from build123d import *

# Parameters (mm, degrees)
F0_W         = 33
F0_H         = 14
F0_R         = 1.75
F1_DEPTH     = 4.8
F2_R         = 1.5
F4_DEPTH     = 4.8
F2_W         = 33
F2_H         = 14
F2_R_2       = 2.5
F2_R_3       = 1.75
F5_DEPTH     = 3.5
F7_DEPTH     = 2.5
F8_W         = 6.5
F8_H         = 5.7518341467
F9_DEPTH     = 12.5
F10_R        = 6
F11_T1_DEPTH = 79.0934091739
F12_R        = 2


# Not quite as in the source:
# - a fillet or chamfer that OpenCascade refuses, or shapes differently, is made with other operations: its cross-section is extruded or revolved along the edge and cut away or added


with BuildPart() as f1:
    # F0 (on Top) → F1 (new body)
    with BuildSketch(Plane.XY):
        with Locations((0, 1.2481658533)):
            Rectangle(F0_W, F0_H)
        with Locations((-13.585, 0)):
            Circle(F0_R, mode=Mode.SUBTRACT)
        with Locations((13.585, 0)):
            Circle(F0_R, mode=Mode.SUBTRACT)
    extrude(amount=F1_DEPTH)

    # F2 (on face) → F4 (cut, through all)
    with BuildSketch(Plane.XY.offset(4.8)):
        with Locations((-7.585, -3)):
            Circle(F2_R)
        with Locations((0, 5)):
            Circle(F2_R)
        with Locations((7.585, -3)):
            Circle(F2_R)
    extrude(amount=-F4_DEPTH, mode=Mode.SUBTRACT)

    # F2 (on face) → F5 (cut)
    with BuildSketch(Plane.XY.offset(4.8)):
        with Locations((0, 1.2481658533)):
            Rectangle(F2_W, F2_H)
        with Locations((-7.585, -3)):
            Circle(F2_R_2, mode=Mode.SUBTRACT)
        with Locations((-13.585, 0)):
            Circle(F2_R_3, mode=Mode.SUBTRACT)
        with Locations((7.585, -3)):
            Circle(F2_R_2, mode=Mode.SUBTRACT)
        with Locations((13.585, 0)):
            Circle(F2_R_3, mode=Mode.SUBTRACT)
        with Locations((0, 5)):
            Circle(F2_R_2, mode=Mode.SUBTRACT)
    extrude(amount=-F5_DEPTH, mode=Mode.SUBTRACT)

    # F6: chamfer of 4 x 2 on 3 edges, made by hand


with BuildPart() as f6_tool2:
    # F6_s3 → F6_t4 (revolve)
    with BuildSketch(Plane.XZ.offset(3)):
        Polygon((-3.085, 1.3), (-5.085, 5.3), (-5.085, 1.3), align=None)
    revolve(axis=Axis((-7.585, -3, 1.3), (0, 0, 1)))

    split(bisect_by=Plane.XZ.offset(5.7518341467), keep=Keep.BOTTOM)

    split(bisect_by=Plane.XY.offset(4.8), keep=Keep.BOTTOM)


with BuildPart() as f1_1:
    add(f1.part)

    # F6_t1: union F6_tool2
    add(f6_tool2.part)


with BuildPart() as f6_tool8:
    # F6_s9 → F6_t10 (revolve)
    with BuildSketch(Plane.XZ.offset(-5)):
        Polygon((4.5, 1.3), (2.5, 5.3), (2.5, 1.3), align=None)
    revolve(axis=Axis((0, 5, 1.3), (0, 0, 1)))

    split(bisect_by=Plane.XZ.offset(-8.2481658533), keep=Keep.TOP)

    split(bisect_by=Plane.XY.offset(4.8), keep=Keep.BOTTOM)


with BuildPart() as f1_2:
    add(f1_1.part)

    # F6_t7: union F6_tool8
    add(f6_tool8.part)


with BuildPart() as f6_tool14:
    # F6_s15 → F6_t16 (revolve)
    with BuildSketch(Plane.XZ.offset(3)):
        Polygon((12.085, 1.3), (10.085, 5.3), (10.085, 1.3), align=None)
    revolve(axis=Axis((7.585, -3, 1.3), (0, 0, 1)))

    split(bisect_by=Plane.XZ.offset(5.7518341467), keep=Keep.BOTTOM)

    split(bisect_by=Plane.XY.offset(4.8), keep=Keep.BOTTOM)


with BuildPart() as f1_3:
    add(f1_2.part)

    # F6_t13: union F6_tool14
    add(f6_tool14.part)

    # F3 (on face) → F7 (cut)
    with BuildSketch(Plane(origin=(0, 0, 0), x_dir=(1, 0, 0), z_dir=(0, 0, -1))):
        Polygon((-5.8818167059, 5.95), (-9.2881832941, 5.95), (-9.4025944029, 5.7518341467), (-5.7674055971, 5.7518341467), align=None)
        Polygon((9.4025944029, 5.7518341467), (5.7674055971, 5.7518341467), (4.1786334118, 3), (5.8818167059, 0.05), (9.2881832941, 0.05), (10.9913665882, 3), align=None)
        Polygon((-1.7031832941, -7.95), (1.7031832941, -7.95), (3.4063665882, -5), (1.7031832941, -2.05), (-1.7031832941, -2.05), (-3.4063665882, -5), align=None)
        Polygon((-5.7674055971, 5.7518341467), (-9.4025944029, 5.7518341467), (-10.9913665882, 3), (-9.2881832941, 0.05), (-5.8818167059, 0.05), (-4.1786334118, 3), align=None)
    extrude(amount=-F7_DEPTH, mode=Mode.SUBTRACT)

    # F8 (on face) → F9 (cut, symmetric)
    with BuildSketch(Plane.XY.offset(1.3)):
        with Locations((-0.835, -2.8759170733)):
            Rectangle(F8_W, F8_H)
    extrude(amount=F9_DEPTH, both=True, mode=Mode.SUBTRACT)

    # F10
    f10_edges = [f1_3.edges().sort_by_distance(p)[0] for p in [
        (-16.5, -5.751834, 0.65),
        (16.5, -5.751834, 0.65),
    ]]
    fillet(f10_edges, radius=F10_R)

    # F11: chamfer of 6 x 15 on 2 edges, made by hand

    # F11_s2 → F11_t1 (cut)
    with BuildSketch(Plane.XY.offset(-38.896704587)):
        Polygon((-1.5, 8.2481658533), (-16.5, 2.2481658533), (-16.5, 8.2481658533), align=None)
        Polygon((16.5, 2.2481658533), (1.5, 8.2481658533), (16.5, 8.2481658533), align=None)
    extrude(amount=F11_T1_DEPTH, mode=Mode.SUBTRACT)

    # F12 (call 1 of 5: OpenCascade refuses the feature's edges together)
    f12_edges = [f1_3.edges().sort_by_distance(p)[0] for p in [
        (-4.085, 0, 0.65),
    ]]
    fillet(f12_edges, radius=F12_R)

    # F12#2 (call 2 of 5)
    f12_2_edges = [f1_3.edges().sort_by_distance(p)[0] for p in [
        (2.415, 0, 0.65),
    ]]
    fillet(f12_2_edges, radius=F12_R)

    # F12#3 (call 3 of 5)
    f12_3_edges = [f1_3.edges().sort_by_distance(p)[0] for p in [
        (2.415, -5.751834, 0.65),
    ]]
    fillet(f12_3_edges, radius=F12_R)

    # F12#4 (call 4 of 5)
    f12_4_edges = [f1_3.edges().sort_by_distance(p)[0] for p in [
        (16.5, 2.248166, 0.65),
    ]]
    fillet(f12_4_edges, radius=F12_R)

    # F12#5 (call 5 of 5)
    f12_5_edges = [f1_3.edges().sort_by_distance(p)[0] for p in [
        (-16.5, 2.248166, 0.65),
    ]]
    fillet(f12_5_edges, radius=F12_R)


solid = f1_3.part
Could you check a few things on this model? Use its own coordinates, in mm. A direction names the side the tool comes from. Give positions to 0.01 mm unless a question says otherwise; leave off trailing zeros. Loops run counter-clockwise (first coordinate to the right, second up) from the corner with the lowest first, then second, coordinate; pieces in that order, holes last. Notation, with made-up numbers: (-11, 56) -> (10, 56) arc R10 cw to (10, 72) -> close; hole circle Ø7 at (5, 17). An arc over 180 degrees is marked (long way). Return JSON: item names as keys, results as strings.
Item 1: If we section it at B-B on z = 0.3: Count the separate pieces of the cut face and the enclosed holes in it, plus the area to 3 significant figures.
Geometry results:
{"separate pieces": "1", "enclosed holes": "3", "area": "211 mm²"}
Item 2: If we section it at A-A on x = 0: List the corners of the cut face in (y, z) for me, plus the area to 3 significant figures.
Geometry results:
{"outline": "(0, 0) -> (2.05, 0) -> (2.05, 2.5) -> (3.5, 2.5) -> (3.5, 4.8) -> (2.25, 4.8) -> (0.5, 1.3) -> (0, 1.3) -> close; (6.5, 2.5) -> (7.95, 2.5) -> (7.95, 0) -> (8.25, 0) -> (8.25, 3.8) -> (7.75, 4.8) -> (6.5, 4.8) -> close", "area": "12.9 mm²"}
Item 3: If we section it at C-C on x = 13: List the corners of the cut face in (y, z) for me, plus the area to 3 significant figures.
Geometry results:
{"outline": "(-5.21, 0) -> (-1.65, 0) -> (-1.65, 1.3) -> (-5.21, 1.3) -> close; (1.65, 0) -> (3.65, 0) -> (3.65, 1.3) -> (1.65, 1.3) -> close", "area": "7.22 mm²"}
Item 4: We'd pull the mould along X, two halves only. Please class faces 4 (the flat face through (0, 7.95, 1)), 5 (the flat face through (8.47, 5.46, 0.85)), 6 (the flat face through (-8.275, 5.538, 0.851)): +X half, -X half, draft (parallel to the pull), parting line (faces both ways), or undercut.
Geometry results:
{"face 4": "undercut", "face 5": "+X half", "face 6": "-X half"}
Item 5: I'm going to push flat-ended pins straight in: pin 1 (1 mm diameter, centred on x = 5, z = 1.5, fed in from +Y); pin 2 (0.6 mm diameter, centred on x = -1.5, z = 0.5, fed in from -Y); pin 3 (2 mm diameter, centred on y = 4, z = 3, fed in from +X). Where does each tip first touch, or does it pass through?
Geometry results:
{"pin 1": "stops at y = 7.03", "pin 2": "stops at y = 0", "pin 3": "stops at x = 4.07"}
Item 6: Which directions (+Z, -Z, +X, -X, +Y, -Y) give clear straight access to the entire face, cutting with the end or side of a thin tool? Please do faces 1 (the flat face through (4.984, -4.395, 1.232)), 2 (the flat face through (2.415, -3, 1)), 3 (the flat face through (-8, -0.05, 1)).
Geometry results:
{"face 1": "-Z", "face 2": "+Z, -Z, -Y", "face 3": "-Z, -Y"}
Item 7: I need wall thicknesses on L1, parallel to X at y = -4, z = 0.3 (3 decimals); L2, parallel to X at y = -2.5, z = 2.65 (3 decimals); L3, parallel to Z at x = -6.5, y = 4.75. Which ranges of each line are inside material? Lowest first, please. Write a range as from..to.
Geometry results:
{"L1": "x = -14.737..-10.414, -4.756..-4.085, 2.43..4.756, 10.414..14.737", "L2": "x = -11.377..-8.999, -6.171..-4.085, 3.793..6.171, 8.999..11.377", "L3": "z = 0..1.3"}
